Read the model definition and answer for the solid it produces. Units are mm, in the model's axes. Give positions to 0.01 mm unless a question says otherwise; leave off trailing zeros. Write each loop counter-clockwise with the first axis right and the second up, starting at its lowest first coordinate (ties: lowest second). Pieces come first, ordered by that corner, then holes. Notation, with made-up numbers: M 2,46 L 35,46 A30 ccw 35,84 Z; hole C 26.5,69 d3. An arc over 180 degrees is marked long. Answer as CSV lines item,"result". Start each with the question number.
```python
from build123d import *

# Parameters (mm, degrees)
F1_DEPTH       = 2
F2_D           = 0.5
F2_CSINK_D     = 1
F2_CSINK_ANGLE = 90
F0_W           = 2.8
F0_H           = 2
F3_DEPTH       = 2


with BuildPart() as f1:
    # F0 (on Front) → F1 (new body)
    with BuildSketch(Plane.XZ):
        Polygon((68.5272171855, 15.8228288673), (-73.0727828145, 15.8228288673), (-73.0727828145, 6.2228288673), (-11.2727828145, 6.2228288673), (-11.2727828145, 8.2228288673), (-11.2727828145, 12.2228288673), (-8.4727828145, 12.2228288673), (-8.4727828145, 8.2228288673), (-8.4727828145, 6.2228288673), (-3.6727828145, 6.2228288673), (-3.6727828145, 8.2228288673), (-3.6727828145, 12.2228288673), (-0.8727828145, 12.2228288673), (-0.8727828145, 8.2228288673), (-0.8727828145, 6.2228288673), (3.9272171855, 6.2228288673), (3.9272171855, 8.2228288673), (3.9272171855, 12.2228288673), (6.7272171855, 12.2228288673), (6.7272171855, 8.2228288673), (6.7272171855, 6.2228288673), (68.5272171855, 6.2228288673), align=None)
    extrude(amount=F1_DEPTH)

    # F2 (through all)
    with Locations(Plane(origin=(0, 0, 0), x_dir=(1, 0, 0), z_dir=(0, 1, 0))):
        with Locations((63.5272171855, -7.2228288673), (44.7272171855, -7.2228288673), (25.9272171855, -7.2228288673), (7.1272171855, -7.2228288673), (-11.6727828145, -7.2228288673), (-30.4727828145, -7.2228288673), (-49.2727828145, -7.2228288673), (-68.0727828145, -7.2228288673)):
            CounterSinkHole(F2_D / 2, F2_CSINK_D / 2, counter_sink_angle=F2_CSINK_ANGLE)

    # F0 (on Front) → F3 (join)
    with BuildSketch(Plane.XZ):
        with Locations((-9.8727828145, 7.2228288673)):
            Rectangle(F0_W, F0_H)
        with Locations((-2.2727828145, 7.2228288673)):
            Rectangle(F0_W, F0_H)
        with Locations((5.3272171855, 7.2228288673)):
            Rectangle(F0_W, F0_H)
    extrude(amount=F3_DEPTH)


solid = f1.part
```
1. Given pin 1 (1.5 mm diameter, centred on x = -49, z = 9, fed in from +Y), flat-ended and moving along its own axis, determine where the tip first touches the part or whether it passes through.
2. Find section B-B on y = -1.3. State how many separate pieces and enclosed holes the cut face has, then the cut area to 3 significant figures.
3. Find section A-A on z = 10.5. Determine the outline of the cut face in (x, y).
4. Find the intervals of material crossed by line 1 (X direction, y = -0.55, z = 9.25); line 2 (Z direction, x = 4, y = -0.55); line 3 (Z direction, x = -11.5, y = -0.15), in increasing order. Write a range as [from, to].
Computed:
1,pin 1,"stops at y = 0"
2,separate pieces,"1"
2,enclosed holes,"11"
2,area,"1,320 mm^2"
3,outline,"M -73.07,-2 L -11.27,-2 L -11.27,0 L -73.07,0 Z; M -8.47,-2 L -3.67,-2 L -3.67,0 L -8.47,0 Z; M -0.87,-2 L 3.93,-2 L 3.93,0 L -0.87,0 Z; M 6.73,-2 L 68.53,-2 L 68.53,0 L 6.73,0 Z"
4,line 1,"x = [-73.07, -11.27], [-8.47, -3.67], [-0.87, 3.93], [6.73, 68.53]"
4,line 2,"z = [6.22, 8.22], [12.22, 15.82]"
4,line 3,"z = [6.22, 6.92], [7.53, 15.82]"
